Source: CAD feature listing. Evaluate the final solid. Frame: model axes, mm. Face numbers are marked on the shaded views. A direction names the side the tool comes from. Round coordinates to 2 decimals unless told otherwise and drop trailing zeros. Loops run counter-clockwise (first coordinate to the right, second up) from the corner with the lowest first, then second, coordinate; pieces in that order, holes last. Notation, with made-up numbers: (29, -7) -> (58, -7) arc R19 ccw to (58, 7) -> close; hole circle Ø6 at (20.25, 9.5). An arc over 180 degrees is marked (long way). Put each result on its own line as item: value. Start each with the question number.
1. Material intervals for L1, parallel to Y at x = 0, z = 10; L2, parallel to Y at x = 10, z = 11.25, sorted ascending.
2. Cut plane A-A (z = 10). Return the cut outline in (x, y).
3. Cut plane B-B (y = 0). Return the cut outline in (x, z) (3 decimals), then the cut area to 3 significant figures.
4. Set-up query: the marked faces 1 and 2. Return all of +Z, -Z, +X, -X, +Y, -Y with unobstructed straight access to the full face (end or side cutting, diameter ignored); none if empty.
5. Draft query along X for the marked faces 3, 4, 5 and 6. Return one class per face: pulls with the +X half, pulls with the -X half, needs draft (parallel to the pull), parting line crosses it, or undercut.
6. Contact query for flat-ended pins moving along their axis: pin 1 (1 mm diameter, centred on x = 5.5, y = -5, fed in from -Z); pin 2 (3 mm diameter, centred on y = 5, z = 10, fed in from +X); pin 3 (1.5 mm diameter, centred on y = 12, z = 7.5, fed in from -X); pin 4 (2 mm diameter, centred on x = -9.5, z = 9, fed in from +Y). Output: stop coordinate, or through.
```python
from build123d import *

# Parameters (mm, degrees)
F0_R     = 15.775
F0_R_2   = 14.5
F0_R_3   = 11.4
F1_DEPTH = 4.3
F2_DEPTH = 13.8
F3_SIZE  = 1.85
F4_R     = 1


with BuildPart() as f1:
    # F0 (on Top) → F1 (new body)
    with BuildSketch(Plane.XY):
        Circle(F0_R)
        Circle(F0_R_2, mode=Mode.SUBTRACT)
        Circle(F0_R_2)
        Circle(F0_R_3, mode=Mode.SUBTRACT)
        Circle(F0_R_3)
    extrude(amount=F1_DEPTH)

    # F0 (on Top) → F2 (join)
    with BuildSketch(Plane.XY):
        Circle(F0_R_2)
        Circle(F0_R_3, mode=Mode.SUBTRACT)
    extrude(amount=F2_DEPTH)

    # F3
    f3_edges = [f1.edges().sort_by_distance(p)[0] for p in [
        (-14.5, 0, 13.8),
    ]]
    chamfer(f3_edges, length=F3_SIZE)

    # F4
    f4_edges = [f1.edges().sort_by_distance(p)[0] for p in [
        (-15.775, 0, 0),
    ]]
    fillet(f4_edges, radius=F4_R)


solid = f1.part
```
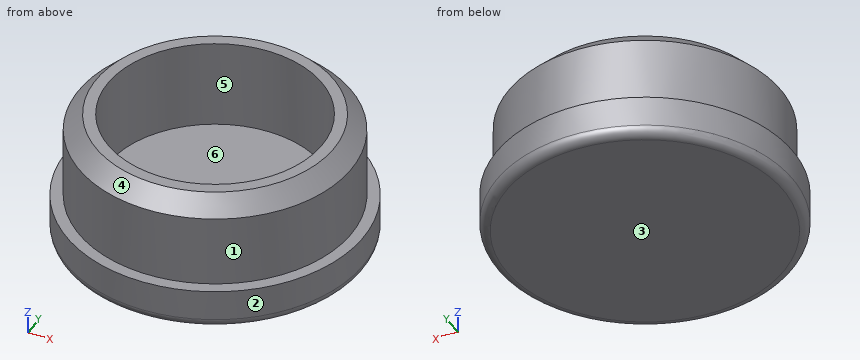
Solution:
1. L1: y = -14.5 to -11.4, 11.4 to 14.5
1. L2: y = -10.5 to -5.47, 5.47 to 10.5
2. outline: circle Ø29 at (0, 0); hole circle Ø22.8 at (0, 0)
3. outline: (-15.775, 1) arc R1 ccw to (-14.775, 0) -> (14.775, 0) arc R1 ccw to (15.775, 1) -> (15.775, 4.3) -> (14.5, 4.3) -> (14.5, 11.95) -> (12.65, 13.8) -> (11.4, 13.8) -> (11.4, 4.3) -> (-11.4, 4.3) -> (-11.4, 13.8) -> (-12.65, 13.8) -> (-14.5, 11.95) -> (-14.5, 4.3) -> (-15.775, 4.3) -> close
3. area: 191 mm^2
4. face 1: +Z
4. face 2: +Z, -Z
5. face 3: needs draft
5. face 4: parting line crosses it
5. face 5: undercut
5. face 6: undercut
6. pin 1: stops at z = 0
6. pin 2: stops at x = 14.07
6. pin 3: stops at x = -9.15
6. pin 4: stops at y = 11.75
